The figure shows three views and two pictorial views of one solid part (mm, origin at its lowest corner). Answer the questions. A direction names the side the tool comes from. Give positions to 0.01 mm unless a question says otherwise; leave off trailing zeros. Loops run counter-clockwise (first coordinate to the right, second up) from the corner with the lowest first, then second, coordinate; pieces in that order, holes last. Notation, with made-up numbers: M -9.5,-19 L 40.5,-19 A31 cw 40.5,19 Z; hole C 73,1 d3. An arc over 180 degrees is marked long. Write item = value, one per line. Start each with the question number.
1. The mould has two halves that part along X. Classify the marked faces 3, 4 and 5: released by +X, released by -X, zero draft, split by the parting line, or undercut.
2. Flat-ended cylindrical pins translate along their axes: pin 1 Ø4 at (y, z) = (4.5, 11.5) entering from +X (1 decimal); pin 2 Ø13 at (x, z) = (41.65, 41.65) entering from -Y; pin 3 Ø8 at (y, z) = (5.5, 48) entering from -X. Find the tip coordinate at first contact, or state that the pin passes through.
3. Section A-A on x = 41.65 is taken. Determine the outline of the cut face in (y, z).
4. For the marked faces 1 and 2, determine the directions among +Z, -Z, +X, -X, +Y, -Y from which every point of the face is accessible in a straight line to the end or side of a thin tool.
5. Consider L1, parallel to X at y = 7.75, z = 41.65; L2, parallel to X at y = 18.25, z = 46.5 (1 decimal); L3, parallel to Y at x = 47.5, z = 71.5. Determine where each line is inside the solid, lowest interval first. Write a range as [from, to].
6. Section B-B on z = 41.65 is taken. Determine the outline of the cut face in (x, y).
7. Section C-C on y = 10.5 is taken. Determine the outline of the cut face in (x, z).
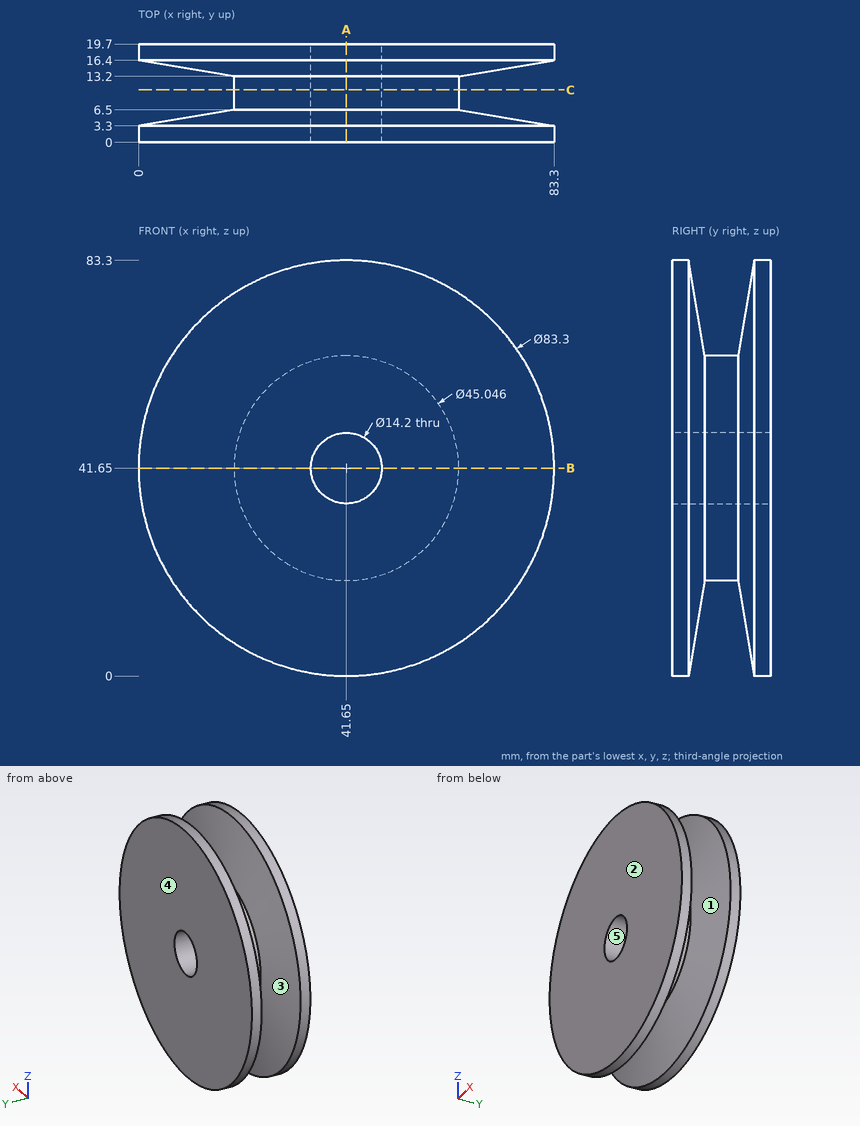
Verdict:
q1.face_3 = split by the parting line
q1.face_4 = zero draft
q1.face_5 = undercut
q2.pin_1 = 72
q2.pin_2 = through
q2.pin_3 = 0.11
q3.outline = M 0,0 L 3.3,0 L 6.5,19.13 L 13.2,19.13 L 16.4,0 L 19.7,0 L 19.7,34.55 L 0,34.55 Z; M 0,48.75 L 19.7,48.75 L 19.7,83.3 L 16.4,83.3 L 13.2,64.17 L 6.5,64.17 L 3.3,83.3 L 0,83.3 Z
q4.face_1 = none
q4.face_2 = +Z, -Z, +X, -X, -Y
q5.L1 = [19.13, 34.55], [48.75, 64.17]
q5.L2 = [0.3, 36.5], [46.8, 83]
q5.L3 = [0, 5.18], [14.52, 19.7]
q6.outline = M 0,0 L 34.55,0 L 34.55,19.7 L 0,19.7 L 0,16.4 L 19.13,13.2 L 19.13,6.5 L 0,3.3 Z; M 48.75,0 L 83.3,0 L 83.3,3.3 L 64.17,6.5 L 64.17,13.2 L 83.3,16.4 L 83.3,19.7 L 48.75,19.7 Z
q7.outline = C 41.65,41.65 d45.05; hole C 41.65,41.65 d14.2
